Geometry: see drawing. Coordinates: mm, zero at the bounding-box minimum. A direction names the side the tool comes from. Coordinates: 2 decimals unless noted, no trailing zeros. Order: outer loops, then holes, each group sorted by start corner. A loop starts at its lowest first (then second) coordinate and runs counter-clockwise, first axis right, second up.
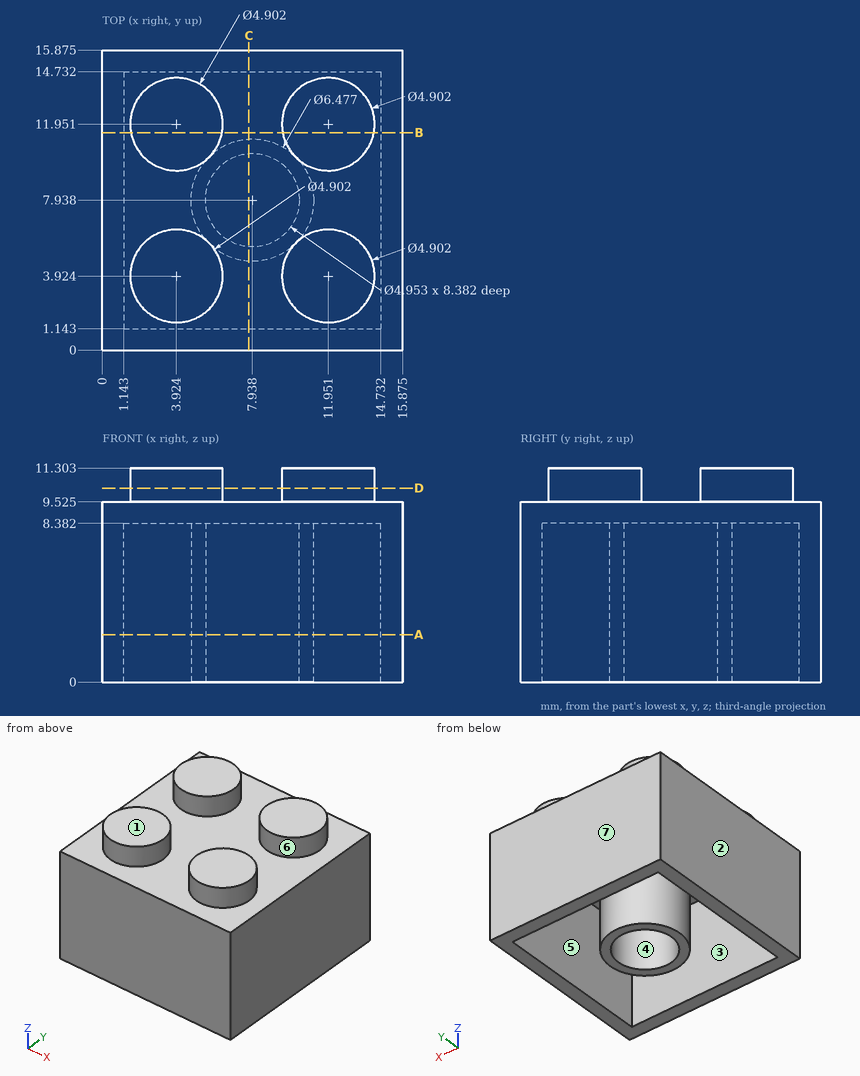
Q1. Material intervals for line 1 along Y through (x, z) = (13.5, 2) (1 decimal); line 2 along Y through (x, z) = (8, 7.75) (1 decimal), sorted ascending.
Solutions:
line 1: y = 0 to 1.1, 14.7 to 15.9
line 2: y = 0 to 1.1, 4.7 to 5.5, 10.4 to 11.2, 14.7 to 15.9
Q2. Pin query (flat end, axial travel): P1, Ø1.5, axis at x = 7, y = 8, coming from the -Z side. Return the tip coordinate at first contact, or that it passes through.
Solutions:
P1: stops at z = 8.38
Q3. Pull-direction query (X, two-part tool) for the marked faces 1, 2, 3 and 4; classes: pulls with the +X half, pulls with the -X half, needs draft (parallel to the pull), parting line crosses it, or undercut.
Solutions:
face 1: needs draft
face 2: pulls with the -X half
face 3: undercut
face 4: undercut
Q4. Section query D-D on z = 10.25. Give the number of separate pieces and of enclosed holes in the cut face.
Solutions:
separate pieces: 4
enclosed holes: 0
Q5. Section query A-A on z = 2.5. Output: boundary loops of the cut face in (x, y) (1 decimal).
Solutions:
outline: (0, 0) - (15.9, 0) - (15.9, 15.9) - (0, 15.9) - close; circle Ø6.5 at (7.9, 7.9); hole (1.1, 1.1) - (14.7, 1.1) - (14.7, 14.7) - (1.1, 14.7) - close; hole circle Ø5 at (7.9, 7.9)
Q6. Section query C-C on x = 7.75. Output: boundary loops of the cut face in (y, z) (1 decimal).
Solutions:
outline: (0, 0) - (1.1, 0) - (1.1, 8.4) - (4.7, 8.4) - (4.7, 0) - (5.5, 0) - (5.5, 8.4) - (10.4, 8.4) - (10.4, 0) - (11.2, 0) - (11.2, 8.4) - (14.7, 8.4) - (14.7, 0) - (15.9, 0) - (15.9, 9.5) - (0, 9.5) - close
Q7. Section query B-B on y = 11.5. Output: boundary loops of the cut face in (x, z) (1 decimal).
Solutions:
outline: (0, 0) - (1.1, 0) - (1.1, 8.4) - (14.7, 8.4) - (14.7, 0) - (15.9, 0) - (15.9, 9.5) - (14.4, 9.5) - (14.4, 11.3) - (9.5, 11.3) - (9.5, 9.5) - (6.3, 9.5) - (6.3, 11.3) - (1.5, 11.3) - (1.5, 9.5) - (0, 9.5) - close
Q8. Set-up query: the marked faces 5, 6 and 7. Return all of +Z, -Z, +X, -X, +Y, -Y with unobstructed straight access to the full face (end or side cutting, diameter ignored); none if empty.
Solutions:
face 5: -Z
face 6: +Z
face 7: +Z, -Z, +X, -X, +Y
